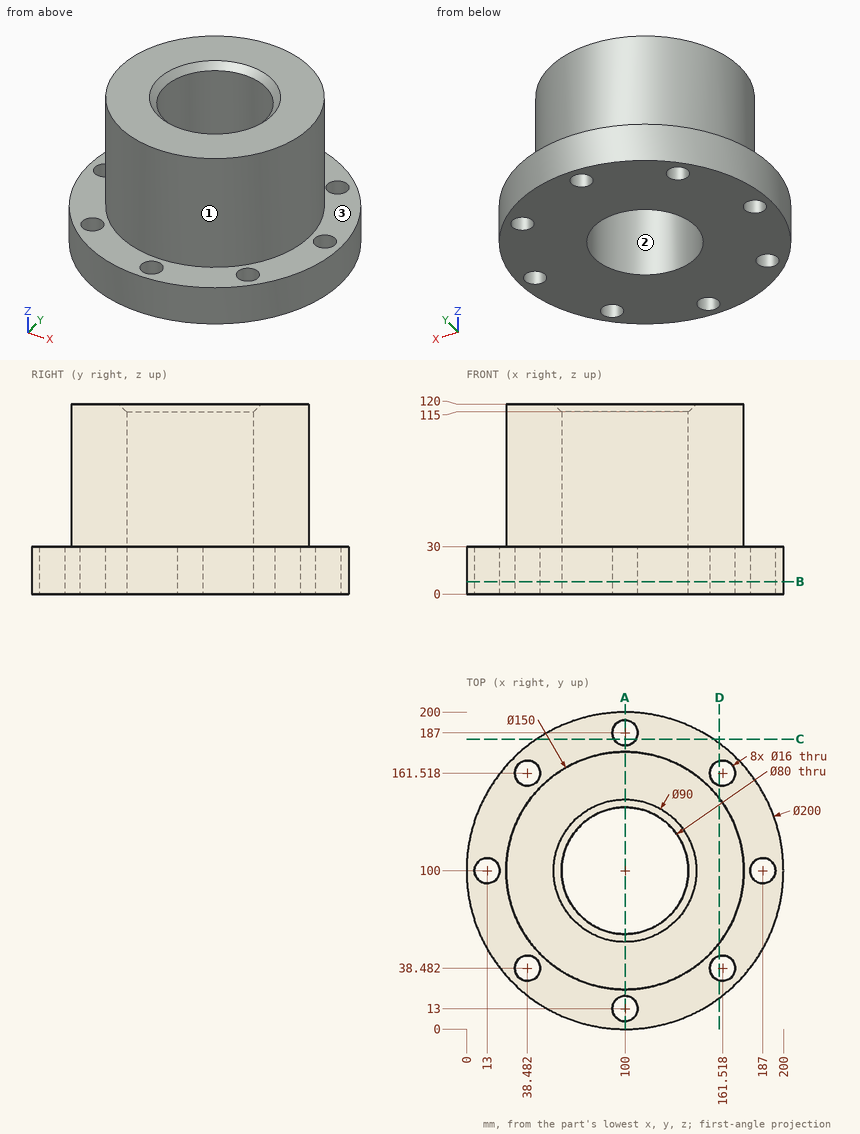
Study the drawing (mm; zero at the part's minimum x, y, z) and answer. Coordinates: 2 decimals unless noted, no trailing zeros. Write each loop counter-clockwise with the first axis right and the second up, starting at its lowest first coordinate (ties: lowest second). Pieces come first, ordered by that corner, then holes. Notation, with made-up numbers: (43, -6) - (71, -6) arc R17 cw to (71, 4) - close; hole circle Ø1 at (15.5, 26.25). An arc over 180 degrees is marked (long way). Return JSON: item names as keys, results as strings. Group by question number.
1. Given pin 1 (2 mm diameter, centred on x = 115, z = 52, fed in from +Y); pin 2 (6 mm diameter, centred on y = 60, z = 69, fed in from -X); pin 3 (21 mm diameter, centred on x = 161.52, y = 38.48, fed in from -Z); pin 4 (18.5 mm diameter, centred on x = 100, y = 13, fed in from +Z), each flat-ended and moving along its own axis, determine where each tip first touches the part or whether it passes through.
2. Determine the mould class of the marked faces 1, 2 and 3 for opening direction Y: released by +Y, released by -Y, zero draft, split by the parting line, or undercut.
3. A cutting plane is placed at B-B, the plane z = 8. Give the number of separate pieces and of enclosed holes in the cut face, plus the area to 3 significant figures.
4. Straight lines are drawn through the part: L1, parallel to Y at x = 100, z = 12; L2, parallel to Y at x = 100, z = 90. For each, find the intervals that lie inside material, in ascending order.
5. A cutting plane is placed at C-C, the plane y = 183. Determine the outline of the cut face in (x, z).
6. A cutting plane is placed at A-A, the plane x = 100. Determine the outline of the cut face in (y, z).
7. A cutting plane is placed at D-D, the plane x = 159.5. Determine the outline of the cut face in (y, z), plus the area to 3 significant figures.
Ans:
{
 "1": {"pin 1": "y = 173.68", "pin 2": "x = 34.76", "pin 3": "z = 0", "pin 4": "z = 30"},
 "2": {"face 1": "split by the parting line", "face 2": "undercut", "face 3": "zero draft"},
 "3": {"separate pieces": "1", "enclosed holes": "9", "area": "24,800 mm²"},
 "4": {"L1": "0 to 5, 21 to 60, 140 to 179, 195 to 200", "L2": "25 to 60, 140 to 175"},
 "5": {"outline": "(44.22, 0) - (93.07, 0) - (93.07, 30) - (44.22, 30) - close; (106.93, 0) - (155.78, 0) - (155.78, 30) - (106.93, 30) - close"},
 "6": {"outline": "(0, 0) - (5, 0) - (5, 30) - (0, 30) - close; (21, 0) - (60, 0) - (60, 115) - (55, 120) - (25, 120) - (25, 30) - (21, 30) - close; (140, 0) - (179, 0) - (179, 30) - (175, 30) - (175, 120) - (145, 120) - (140, 115) - close; (195, 0) - (200, 0) - (200, 30) - (195, 30) - close"},
 "7": {"outline": "(19.63, 0) - (30.74, 0) - (30.74, 30) - (19.63, 30) - close; (46.22, 0) - (153.78, 0) - (153.78, 30) - (145.66, 30) - (145.66, 120) - (54.34, 120) - (54.34, 30) - (46.22, 30) - close; (169.26, 0) - (180.37, 0) - (180.37, 30) - (169.26, 30) - close", "area": "12,100 mm²"}
}
